Check sheet for the modelled part. Datum: model origin and axes. Units: mm. A direction names the side the tool comes from. Round coordinates to 2 decimals unless told otherwise and drop trailing zeros. Write each loop counter-clockwise with the first axis right and the second up, starting at its lowest first coordinate (ties: lowest second). Pieces come first, ordered by that corner, then holes. Notation, with made-up numbers: (34.5, 78) -> (52.5, 78) arc R21 cw to (52.5, 112) -> close; hole circle Ø6 at (51, 63.25). An arc over 180 degrees is marked (long way). One line per item, written item: value.
from build123d import *

# Parameters (mm, degrees)
SKETCH_1_W               = 25
SKETCH_1_H               = 30
EXTRUDE_1_DEPTH          = 200
SKETCH_2_OUTSIDE_W       = 107.38
SKETCH_2_OUTSIDE_H       = 112.38
SKETCH_2_OUTSIDE_W_2     = 25
SKETCH_2_OUTSIDE_H_2     = 30
SKETCH_2_OUTSIDE_W_3     = 23
SKETCH_2_OUTSIDE_H_3     = 28
CUT_EXTRUDE_1_DEPTH      = 200
SKETCH_3_R               = 2.025
CUT_EXTRUDE_2_DEPTH      = 31
SKETCH_4_R               = 1.525
CUT_EXTRUDE_3_DEPTH      = 1
CUT_EXTRUDE_3_DEPTH_BACK = 26
SKETCH_5_R               = 1.525
CUT_EXTRUDE_4_DEPTH      = 1
CUT_EXTRUDE_4_DEPTH_BACK = 26
SKETCH_6_R               = 3
CUT_EXTRUDE_5_DEPTH      = 5
SKETCH_7_R               = 3
CUT_EXTRUDE_6_DEPTH      = 5
CUT_EXTRUDE_START        = -31
CUT_EXTRUDE_7_DEPTH      = 32
PATTERN_LINEAR_1_COUNT   = 8
PATTERN_LINEAR_1_PITCH   = 45
SKETCH_10_R              = 1.525
CUT_EXTRUDE_9_DEPTH      = 31
SKETCH_11_R              = 1.525
CUT_EXTRUDE_10_DEPTH     = 3


with BuildPart() as part:
    # 草图1 → 凸台-拉伸1 (new body, symmetric)
    with BuildSketch(Plane.XY):
        Rectangle(SKETCH_1_W, SKETCH_1_H)
    extrude(amount=EXTRUDE_1_DEPTH, both=True)

    # 草图2 outside → 切除-拉伸1 (cut, symmetric)
    with BuildSketch(Plane.XY):
        Rectangle(SKETCH_2_OUTSIDE_W, SKETCH_2_OUTSIDE_H)
        Rectangle(SKETCH_2_OUTSIDE_W_2, SKETCH_2_OUTSIDE_H_2, mode=Mode.SUBTRACT)
        Rectangle(SKETCH_2_OUTSIDE_W_3, SKETCH_2_OUTSIDE_H_3)
    extrude(amount=CUT_EXTRUDE_1_DEPTH, both=True, mode=Mode.SUBTRACT)

    # 草图3 → 切除-拉伸2 (cut, through all)
    with BuildSketch(Plane(origin=(0, 15, 0), x_dir=(1, 0, 0), z_dir=(0, 1, 0))):
        with Locations((0, 172.5)):
            Circle(SKETCH_3_R)
        with Locations((0, 192.5)):
            Circle(SKETCH_3_R)
    extrude(amount=-CUT_EXTRUDE_2_DEPTH, mode=Mode.SUBTRACT)

    # 草图4 → 切除-拉伸3 (cut, two sides)
    with BuildSketch(Plane(origin=(12.5, 0, 0), x_dir=(0, 0, -1), z_dir=(1, 0, 0))) as cut_extrude_3_sk:
        with Locations((-170, -9.5)):
            Circle(SKETCH_4_R)
        with Locations((-189, -9.5)):
            Circle(SKETCH_4_R)
        with Locations((-189, 9.5)):
            Circle(SKETCH_4_R)
        with Locations((-170, 9.5)):
            Circle(SKETCH_4_R)
    extrude(amount=CUT_EXTRUDE_3_DEPTH, mode=Mode.SUBTRACT)
    extrude(cut_extrude_3_sk.sketch, amount=-CUT_EXTRUDE_3_DEPTH_BACK, mode=Mode.SUBTRACT)

    # 草图5 → 切除-拉伸4 (cut, two sides)
    with BuildSketch(Plane(origin=(12.5, 0, 0), x_dir=(0, 0, -1), z_dir=(1, 0, 0))) as cut_extrude_4_sk:
        with Locations((-95, 9.5)):
            Circle(SKETCH_5_R)
        with Locations((-114, 9.5)):
            Circle(SKETCH_5_R)
        with Locations((-114, -9.5)):
            Circle(SKETCH_5_R)
        with Locations((-95, -9.5)):
            Circle(SKETCH_5_R)
    extrude(amount=CUT_EXTRUDE_4_DEPTH, mode=Mode.SUBTRACT)
    extrude(cut_extrude_4_sk.sketch, amount=-CUT_EXTRUDE_4_DEPTH_BACK, mode=Mode.SUBTRACT)

    # 草图6 → 切除-拉伸5 (cut)
    with BuildSketch(Plane(origin=(12.5, 0, 0), x_dir=(0, 0, -1), z_dir=(1, 0, 0))):
        with Locations((-170, 9.5)):
            Circle(SKETCH_6_R)
        with Locations((-170, -9.5)):
            Circle(SKETCH_6_R)
        with Locations((-189, -9.5)):
            Circle(SKETCH_6_R)
        with Locations((-189, 9.5)):
            Circle(SKETCH_6_R)
    extrude(amount=-CUT_EXTRUDE_5_DEPTH, mode=Mode.SUBTRACT)

    # 草图7 → 切除-拉伸6 (cut)
    with BuildSketch(Plane(origin=(12.5, 0, 0), x_dir=(0, 0, -1), z_dir=(1, 0, 0))):
        with Locations((-114, 9.5)):
            Circle(SKETCH_7_R)
        with Locations((-95, 9.5)):
            Circle(SKETCH_7_R)
        with Locations((-95, -9.5)):
            Circle(SKETCH_7_R)
        with Locations((-114, -9.5)):
            Circle(SKETCH_7_R)
    extrude(amount=-CUT_EXTRUDE_6_DEPTH, mode=Mode.SUBTRACT)

    # 草图8 → 切除-拉伸7 (cut)
    with BuildSketch(Plane(origin=(0, 15, 0), x_dir=(1, 0, 0), z_dir=(0, 1, 0)).offset(CUT_EXTRUDE_START)):
        with BuildLine():
            Line((-6, -172.5), (-6, -167.5))
            ThreePointArc((-6, -167.5), (0, -161.5), (6, -167.5))
            Line((6, -167.5), (6, -172.5))
            ThreePointArc((6, -172.5), (0, -178.5), (-6, -172.5))
        make_face()
    cut_extrude_7 = extrude(amount=CUT_EXTRUDE_7_DEPTH, mode=Mode.SUBTRACT)

    # 阵列(线性)1: 切除-拉伸7 ×8
    with Locations(*[(0, 0, -i * PATTERN_LINEAR_1_PITCH) for i in range(1, PATTERN_LINEAR_1_COUNT)]):
        add(cut_extrude_7, mode=Mode.SUBTRACT)

    # 草图10 → 切除-拉伸9 (cut, through all)
    with BuildSketch(Plane(origin=(0, 15, 0), x_dir=(1, 0, 0), z_dir=(0, 1, 0))):
        with Locations((8.5, 112.5)):
            Circle(SKETCH_10_R)
        with Locations((8.5, 132.5)):
            Circle(SKETCH_10_R)
    extrude(amount=-CUT_EXTRUDE_9_DEPTH, mode=Mode.SUBTRACT)

    # 草图11 → 切除-拉伸10 (cut)
    with BuildSketch(Plane(origin=(12.5, 0, 0), x_dir=(0, 0, -1), z_dir=(1, 0, 0))):
        with Locations((122.5, 10.999999999)):
            Circle(SKETCH_11_R)
        with Locations((102.5, 10.999999999)):
            Circle(SKETCH_11_R)
        with Locations((102.5, -11)):
            Circle(SKETCH_11_R)
        with Locations((122.5, -11)):
            Circle(SKETCH_11_R)
    extrude(amount=-CUT_EXTRUDE_10_DEPTH, mode=Mode.SUBTRACT)


solid = part.part
Item 1: Release check for a two-part mould opening along Y. For faces 1 (the flat face through (11.5, 0, 3)), 2 (the flat face through (0, -15, 3)), 3 (the flat face through (12.5, 0, 3)) record: pulls with the +Y half, pulls with the -Y half, needs draft (parallel to the pull), parting line crosses it, or undercut.
Result set:
face 1: undercut
face 2: pulls with the -Y half
face 3: needs draft
Item 2: Sectioned sample at B-B (z = 148). Enter the section's corners in (x, y), then the cut area to 3 significant figures.
Result set:
outline: (-12.5, -15) -> (12.5, -15) -> (12.5, 15) -> (-12.5, 15) -> close; hole (-11.5, -14) -> (11.5, -14) -> (11.5, 14) -> (-11.5, 14) -> close
area: 106 mm^2
Item 3: Material ranges on line 1 along Y through (x, z) = (12.3, 95); line 2 along X through (y, z) = (-3.25, -148.5); line 3 along Y through (x, z) = (6, -2.5), recorded low to high.
Result set:
line 1: -15 to -12.5, -6.5 to 6.5, 12.5 to 15
line 2: -12.5 to -11.5, 11.5 to 12.5
line 3: -15 to -14, 14 to 15
Item 4: Sectioned sample at A-A (y = -3). Enter the section's corners in (x, z).
Result set:
outline: (-12.5, -200) -> (-11.5, -200) -> (-11.5, 200) -> (-12.5, 200) -> close; (11.5, -200) -> (12.5, -200) -> (12.5, 200) -> (11.5, 200) -> close
Item 5: Tool access check on faces 4 (the flat face through (0, 14, 3)), 5 (the flat face through (-12, 0, -200)). Record the directions out of +Z, -Z, +X, -X, +Y, -Y that give a thin tool (end or side, any length) a straight path to the whole face; none if there is none.
Result set:
face 4: +Z, -Z
face 5: -Z, +X, -X, +Y, -Y
